The listing builds one solid part. Answer for the finished solid, in the listing's coordinates (mm). A direction names the side the tool comes from. Round coordinates to 2 decimals unless told otherwise and drop trailing zeros. Order: outer loops, then holes, each group sorted by start corner. A loop starts at its lowest first (then second) coordinate and runs counter-clockwise, first axis right, second up. Notation, with made-up numbers: (21.5, 35) - (44.5, 35) arc R11 cw to (44.5, 53) - close; hole circle Ø11 at (42.5, -12.5). An arc over 180 degrees is marked (long way). One line per item, written item: value. Start each with the question number.
1. Flat-ended cylindrical pins translate along their axes: P1, Ø2, axis at x = -1.5, y = -1.5, coming from the -Z side; P2, Ø0.6, axis at x = 0, z = 1.5, coming from the -Y side; P3, Ø0.7, axis at y = -0.5, z = 1.5, coming from the +X side; P4, Ø0.9, axis at x = -1, z = 1.5, coming from the +Y side. Find the tip coordinate at first contact, or state that the pin passes through.
2. Section A-A, the plane z = -5 is taken. Give the vertices of the cut face in (x, y), then the cut area to 3 significant figures.
3. For a pull along X with two mould halves and no side action, classify faces 3 (the flat face through (0, 0, -8)), 4 (the cylindrical face through (-0.86, 2.08, 0.24)), 5 (the flat face through (0.26, -1, 1)) as released by +X, released by -X, zero draft, split by the parting line, or undercut.
4. A tool of negligible diameter and unlimited length cuts with its end or side. For faces 1 (the flat face through (-1, 1, 0)), 2 (the flat face through (1, -0.26, 1)), from which of +Z, -Z, +X, -X, +Y, -Y can it reach the whole face along a straight path? Write none if from no direction.
5. Straight lines are drawn through the part: line 1 (X direction, y = 0, z = -6); line 2 (Z direction, x = 1.5, y = -0.15); line 3 (Y direction, x = -0.75, z = -0.25). For each, find the intervals that lie inside material, in ascending order.
from build123d import *

# Parameters (mm, degrees)
CUT_EXTRUDE2_DEPTH = 0.85
FILLET1_R          = 1
CHAMFER1_SIZE      = 0.225
ESQUISSE1_R        = 1.25
BOSS_EXTRU_1_DEPTH = 8


with BuildPart() as part:
    # Sketch1 → Revolve1 (revolve)
    with BuildSketch(Plane(origin=(0, 0, 0), x_dir=(0, 0, -1), z_dir=(1, 0, 0))):
        with BuildLine():
            Line((-1.133333333, 2.25), (0, 2.25))
            Line((0, 2.25), (0, 1.25))
            Line((0, 1.25), (4, 1.25))
            Line((4, 1.25), (4, 0))
            Line((4, 0), (-1.7, 0))
            ThreePointArc((-1.7, 0), (-1.556155418, 1.1601305), (-1.133333333, 2.25))
        make_face()
    revolve(axis=Axis((0, 0, 33.735969773), (0, 0, -1)))

    # Sketch2 → Cut-Extrude2 (cut)
    with BuildSketch(Plane(origin=(0, 0, 1.7), x_dir=(-1, 0, 0), z_dir=(0, 0, -1))):
        Polygon((0, 1.3), (0.26, 1.3), (0.26, 0.26), (1.3, 0.26), (1.3, 0), (1.3, -0.26), (0.26, -0.26), (0.26, -1.3), (0, -1.3), (-0.26, -1.3), (-0.26, -0.26), (-1.3, -0.26), (-1.3, 0), (-1.3, 0.26), (-0.26, 0.26), (-0.26, 1.3), align=None)
    extrude(amount=CUT_EXTRUDE2_DEPTH, mode=Mode.SUBTRACT)

    # Fillet1
    fillet1_edges = [part.edges().sort_by_distance(p)[0] for p in [
        (0, -2.25, 1.133333333),
    ]]
    fillet(fillet1_edges, radius=FILLET1_R)

    # Chamfer1
    chamfer1_edges = [part.edges().sort_by_distance(p)[0] for p in [
        (0, -1.25, -4),
    ]]
    chamfer(chamfer1_edges, length=CHAMFER1_SIZE)

    # Esquisse1 → Boss.-Extru.1 (add)
    with BuildSketch(Plane(origin=(0, 0, 0), x_dir=(-1, 0, 0), z_dir=(0, 0, -1))):
        Circle(ESQUISSE1_R)
    extrude(amount=BOSS_EXTRU_1_DEPTH)


solid = part.part
Answer list:
1. P1: stops at z = -8
1. P2: stops at y = -1.95
1. P3: stops at x = 1.94
1. P4: stops at y = 1.88
2. outline: circle Ø2.5 at (0, 0)
2. area: 4.91 mm²
3. face 3: zero draft
3. face 4: split by the parting line
3. face 5: undercut
4. face 1: -Z
4. face 2: +Z
5. line 1: x = -1.25 to 1.25
5. line 2: z = 0 to 1.45
5. line 3: y = -1 to 1
